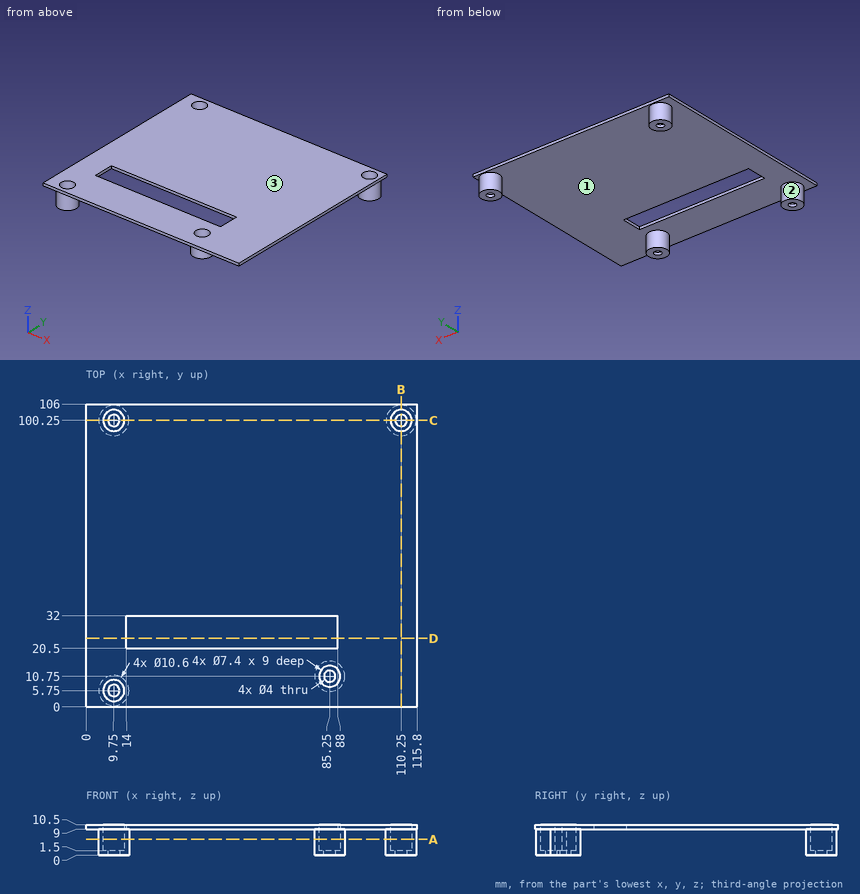
Here's the drawing with two shaded views (mm, measured from the low corner). I have some questions. Give positions to 0.01 mm unless a question says otherwise; leave off trailing zeros. Loops run counter-clockwise (first coordinate to the right, second up) from the corner with the lowest first, then second, coordinate; pieces in that order, holes last. Notation, with made-up numbers: (-15.5, -11.75) -> (35.5, -11.75) arc R27 cw to (35.5, 7.25) -> close; hole circle Ø2 at (-19, 52.5). An arc over 180 degrees is marked (long way). Use one line per item in the form item = value.
1) We'd pull the mould along X, two halves only. Please class the marked faces 1, 2 and 3: released by +X, released by -X, zero draft, split by the parting line, or undercut.
Answers:
face_1 = undercut
face_2 = undercut
face_3 = zero draft
2) If we section it at A-A (z = 5.5): Please give me the cut outline in (x, y), plus the area to 3 significant figures.
Answers:
outline = circle Ø10.6 at (9.75, 5.75); circle Ø10.6 at (9.75, 100.25); circle Ø10.6 at (85.25, 10.75); circle Ø10.6 at (110.25, 100.25); hole circle Ø7.4 at (9.75, 5.75); hole circle Ø7.4 at (9.75, 100.25); hole circle Ø7.4 at (85.25, 10.75); hole circle Ø7.4 at (110.25, 100.25)
area = 181 mm²
3) If we section it at C-C (y = 100.25): Please give me the cut outline in (x, z), plus the area to 3 significant figures.
Answers:
outline = (0, 9) -> (4.45, 9) -> (4.45, 0) -> (7.75, 0) -> (7.75, 1.5) -> (6.05, 1.5) -> (6.05, 10.5) -> (0, 10.5) -> close; (11.75, 0) -> (15.05, 0) -> (15.05, 9) -> (104.95, 9) -> (104.95, 0) -> (108.25, 0) -> (108.25, 1.5) -> (106.55, 1.5) -> (106.55, 10.5) -> (13.45, 10.5) -> (13.45, 1.5) -> (11.75, 1.5) -> close; (112.25, 0) -> (115.55, 0) -> (115.55, 9) -> (115.8, 9) -> (115.8, 10.5) -> (113.95, 10.5) -> (113.95, 1.5) -> (112.25, 1.5) -> close
area = 219 mm²
4) If we section it at D-D (y = 24): Please give me the cut outline in (x, z), plus the area to 3 significant figures.
Answers:
outline = (0, 9) -> (14, 9) -> (14, 10.5) -> (0, 10.5) -> close; (88, 9) -> (115.8, 9) -> (115.8, 10.5) -> (88, 10.5) -> close
area = 62.7 mm²
5) I need wall thicknesses on line 1 along Y through (x, z) = (9.75, 0.7); line 2 along X through (y, z) = (98, 8); line 3 along Y through (x, z) = (23.5, 9.5). Which ranges of each line are inside material? Lowest first, please.
Answers:
line_1 = 0.45 to 3.75, 7.75 to 11.05, 94.95 to 98.25, 102.25 to 105.55
line_2 = 4.95 to 6.81, 12.69 to 14.55, 105.45 to 107.31, 113.19 to 115.05
line_3 = 0 to 20.5, 32 to 106
6) If we section it at B-B (x = 110.25): Please give me the cut outline in (y, z), plus the area to 3 significant figures.
Answers:
outline = (0, 9) -> (94.95, 9) -> (94.95, 0) -> (98.25, 0) -> (98.25, 1.5) -> (96.55, 1.5) -> (96.55, 10.5) -> (0, 10.5) -> close; (102.25, 0) -> (105.55, 0) -> (105.55, 9) -> (106, 9) -> (106, 10.5) -> (103.95, 10.5) -> (103.95, 1.5) -> (102.25, 1.5) -> close
area = 182 mm²
7) Will these pins go through, and if not, where does the flat tip stop? pin 1 (12 mm diameter, centred on x = 38, y = 37.5, fed in from -Z); pin 2 (4.5 mm diameter, centred on x = 9.75, y = 5.75, fed in from +Z); pin 3 (1.5 mm diameter, centred on x = 90.5, z = 2.5, fed in from +Y).
Answers:
pin_1 = 9
pin_2 = 1.5
pin_3 = 13.55
